Check sheet for the modelled part. Datum: model origin and axes. Units: mm. A direction names the side the tool comes from. Round coordinates to 2 decimals unless told otherwise and drop trailing zeros. Loops run counter-clockwise (first coordinate to the right, second up) from the corner with the lowest first, then second, coordinate; pieces in that order, holes last. Notation, with made-up numbers: (7, 22) -> (47, 22) arc R25 cw to (47, 58) -> close; hole circle Ø11 at (50, 26). An arc over 180 degrees is marked (long way). Use one line per item in the form item = value. Start each with the question number.
(1) Sectioned sample at A-A (z = -22.5). Record the cut outline in (x, y).
(2) Material ranges on probe 1 along Z at (x, y) = (2.55, 5.5); probe 2 along Z at (x, y) = (2.2, 5.25); probe 3 along X at (y, z) = (4.25, -12.5), recorded low to high. Write a range as [from, to].
(3) Set-up check for faces 4 (the flat face through (3, 6, 28.501)), 5 (the flat face through (0.6, 6, -20)): record each of +Z, -Z, +X, -X, +Y, -Y from which the full face is reachable in a straight line by a thin tool's end or side.
(4) Draft check along Z on faces 1 (the flat face through (0.6, 6, 24)), 2 (the flat face through (0, 6, -19)), 3 (the flat face through (2, 6, -36.499)). Enter one of: released by +Z, released by -Z, zero draft, split by the parting line, or undercut.
(5) Go/stop test with flat-tipped pins: pin 1 (0.5 mm diameter, centred on x = 0, y = 5, fed in from +Z); pin 2 (0.6 mm diameter, centred on y = 4.5, z = -27.5, fed in from -X); pin 3 (0.7 mm diameter, centred on x = 0.5, y = 7, fed in from +Z). Record where each tip stops, or that it passes through.
from build123d import *

# Parameters (mm, degrees)
SKETCH_1_W          = 65
SKETCH_1_H          = 6
SKETCH_1_R          = 0.75
EXTRUDE_1_DEPTH     = 5
SKETCH_2_W          = 0.6
SKETCH_2_H          = 1.22
SKETCH_2_H_2        = 0.34
CUT_EXTRUDE_1_DEPTH = 15


with BuildPart() as part:
    # Sketch 1 → Extrude 1 (new body)
    with BuildSketch(Plane(origin=(0, 0, 0), x_dir=(0, 0, -1), z_dir=(1, 0, 0))):
        with Locations((3.998772772, 5.663725322)):
            Rectangle(SKETCH_1_W, SKETCH_1_H)
        with Locations((-6.001227228, 5.663725322)):
            Circle(SKETCH_1_R, mode=Mode.SUBTRACT)
        with Locations((13.998772772, 5.663725322)):
            Circle(SKETCH_1_R, mode=Mode.SUBTRACT)
    extrude(amount=EXTRUDE_1_DEPTH)

    # Sketch 2 → Cut-Extrude 1 (cut)
    with BuildSketch(Plane(origin=(0, 8.663725322, 0), x_dir=(1, 0, 0), z_dir=(0, 1, 0))):
        with Locations((0.3, 34.668772772)):
            Rectangle(SKETCH_2_W, SKETCH_2_H)
        with Locations((0.3, 32.228772772)):
            Rectangle(SKETCH_2_W, SKETCH_2_H)
        with Locations((0.3, 29.788772772)):
            Rectangle(SKETCH_2_W, SKETCH_2_H)
        with Locations((0.3, 27.348772772)):
            Rectangle(SKETCH_2_W, SKETCH_2_H)
        with Locations((0.3, 24.908772772)):
            Rectangle(SKETCH_2_W, SKETCH_2_H)
        with Locations((0.3, 22.468772772)):
            Rectangle(SKETCH_2_W, SKETCH_2_H)
        with Locations((0.3, 20.028772772)):
            Rectangle(SKETCH_2_W, SKETCH_2_H)
        with Locations((0.3, 17.588772772)):
            Rectangle(SKETCH_2_W, SKETCH_2_H)
        with Locations((0.3, 15.148772772)):
            Rectangle(SKETCH_2_W, SKETCH_2_H)
        with Locations((0.3, 12.708772772)):
            Rectangle(SKETCH_2_W, SKETCH_2_H)
        with Locations((0.3, 10.268772772)):
            Rectangle(SKETCH_2_W, SKETCH_2_H)
        with Locations((0.3, 7.828772772)):
            Rectangle(SKETCH_2_W, SKETCH_2_H)
        with Locations((0.3, 5.388772772)):
            Rectangle(SKETCH_2_W, SKETCH_2_H)
        with Locations((0.3, 2.948772772)):
            Rectangle(SKETCH_2_W, SKETCH_2_H)
        with Locations((0.3, 0.508772772)):
            Rectangle(SKETCH_2_W, SKETCH_2_H)
        with Locations((0.3, -1.931227228)):
            Rectangle(SKETCH_2_W, SKETCH_2_H)
        with Locations((0.3, -4.371227228)):
            Rectangle(SKETCH_2_W, SKETCH_2_H)
        with Locations((0.3, -6.811227228)):
            Rectangle(SKETCH_2_W, SKETCH_2_H)
        with Locations((0.3, -9.251227228)):
            Rectangle(SKETCH_2_W, SKETCH_2_H)
        with Locations((0.3, -11.691227228)):
            Rectangle(SKETCH_2_W, SKETCH_2_H)
        with Locations((0.3, -14.131227228)):
            Rectangle(SKETCH_2_W, SKETCH_2_H)
        with Locations((0.3, -16.571227228)):
            Rectangle(SKETCH_2_W, SKETCH_2_H)
        with Locations((0.3, -19.011227228)):
            Rectangle(SKETCH_2_W, SKETCH_2_H)
        with Locations((0.3, -21.451227228)):
            Rectangle(SKETCH_2_W, SKETCH_2_H)
        with Locations((0.3, -23.891227228)):
            Rectangle(SKETCH_2_W, SKETCH_2_H)
        with Locations((0.3, -26.331227228)):
            Rectangle(SKETCH_2_W, SKETCH_2_H)
        with Locations((0.3, -28.331227228)):
            Rectangle(SKETCH_2_W, SKETCH_2_H_2)
    extrude(amount=-CUT_EXTRUDE_1_DEPTH, mode=Mode.SUBTRACT)


solid = part.part
Checks:
q1.outline = (0.6, 2.66) -> (5, 2.66) -> (5, 8.66) -> (0.6, 8.66) -> close
q2.probe_1 = [-36.5, -14.73], [-13.27, 5.27], [6.73, 28.5]
q2.probe_2 = [-36.5, -14.62], [-13.37, 5.38], [6.63, 28.5]
q2.probe_3 = [0.6, 5]
q3.face_4 = +Z, +X, -X, +Y, -Y
q3.face_5 = -X, +Y, -Y
q4.face_1 = undercut
q4.face_2 = zero draft
q4.face_3 = released by -Z
q5.pin_1 = 28.16
q5.pin_2 = 0.6
q5.pin_3 = 28.5
